CAD build for the part. Positions are in the model's coordinates, mm. Give positions to 0.01 mm unless a question says otherwise; leave off trailing zeros. Loops run counter-clockwise (first coordinate to the right, second up) from the corner with the lowest first, then second, coordinate; pieces in that order, holes last.
Autodesk Inventor part; units mm, degrees
ref_plane "YZ Plane" through (0, 0, 0) normal (1, 0, 0) x (0, 1, 0)
ref_plane "XZ Plane" through (0, 0, 0) normal (0, 1, 0) x (-1, 0, 0)
ref_plane "XY Plane" through (0, 0, 0) normal (0, 0, 1) x (1, 0, 0)
sketch "Sketch1" plane through (0, 0, 0) normal (0, 0, 1) x (1, 0, 0)
  line L0 (-76.2, 25.4) -> (76.2, 25.4) construction
  line L1 (76.2, 25.4) -> (76.2, -25.4) construction
  line L2 (76.2, -25.4) -> (-76.2, -25.4) construction
  line L3 (-76.2, -25.4) -> (-76.2, 25.4) construction
  line L4 (-76.2, 25.4) -> (76.2, -25.4) construction
  line L5 (76.2, 25.4) -> (-76.2, -25.4) construction
  line L6 (63.5, 17.4625) -> (63.5, -17.4625) construction
  line L7 (9.525, 15.875) -> (41.275, 15.875) construction
  line L8 (41.275, 15.875) -> (41.275, -15.875) construction
  line L9 (41.275, -15.875) -> (9.525, -15.875) construction
  line L10 (9.525, -15.875) -> (9.525, 15.875) construction
  line L11 (9.525, 15.875) -> (41.275, -15.875) construction
  line L12 (41.275, 15.875) -> (9.525, -15.875) construction
  line L13 (76.2, 101.6) -> (187.452, 101.6) construction
  line L14 (187.452, 101.6) -> (187.452, -25.4) construction
  line L15 (187.452, -25.4) -> (76.2, -25.4) construction
  line L16 (76.2, -25.4) -> (76.2, 101.6) construction
  line L17 (76.2, 101.6) -> (187.452, -25.4) construction
  line L18 (187.452, 101.6) -> (76.2, -25.4) construction
  point P0 (0, 0)
  point P1 (63.5, 0)
  point P2 (25.4, 0)
  point P3 (50.8, 0)
  point P4 (0, 0)
  point P5 (9.525, 0)
  point P6 (-12.7, 17.4625)
  point P7 (-12.7, -17.4625)
  point P8 (-25.4, 0)
  point P9 (-38.1, 17.4625)
  point P10 (-38.1, -17.4625)
  point P11 (-50.8, 0)
  point P12 (-63.5, 17.4625)
  point P13 (-63.5, -17.4625)
  point P14 (131.826, 38.1)
  dimension "d0" = 152.4
  dimension "d1" = 50.8
  dimension "d2" = 34.925
  dimension "d3" = 12.7
  dimension "d4" = 31.75
  dimension "d5" = 31.75
  dimension "d6" = 34.925
  dimension "d7" = 25.4
  dimension "d8" = 9.525
  dimension "d9" = 12.7
  dimension "d10" = 12.7
  dimension "d11" = 12.7
  dimension "d12" = 12.7
  dimension "d13" = 12.7
  dimension "d14" = 111.252
  dimension "d15" = 127
  dimension "d16" = 76.2
sketch "Sketch2" plane through (0, 0, 0) normal (0, 0, 1) x (1, 0, 0)
  line L0 (63.5, 17.4625) -> (63.5, -17.4625) construction
  line L1 (76.2, 25.4) -> (76.2, -25.4) construction
  line L2 (76.2, -25.4) -> (76.2, 101.6) construction
  line L3 (187.452, -25.4) -> (76.2, -25.4) construction
  line L4 (187.452, 101.6) -> (187.452, -25.4) construction
  line L5 (76.2, 101.6) -> (187.452, -25.4) construction
  line L6 (187.452, 101.6) -> (76.2, -25.4) construction
  line L7 (76.2, 101.6) -> (187.452, 101.6) construction
  line L8 (9.525, 15.875) -> (41.275, 15.875) construction
  line L9 (41.275, 15.875) -> (41.275, -15.875) construction
  line L10 (41.275, -15.875) -> (9.525, -15.875) construction
  line L11 (9.525, -15.875) -> (9.525, 15.875) construction
  line L12 (9.525, 15.875) -> (41.275, -15.875) construction
  line L13 (41.275, 15.875) -> (9.525, -15.875) construction
  line L14 (-76.2, 25.4) -> (76.2, 25.4) construction
  line L15 (76.2, -25.4) -> (-76.2, -25.4) construction
  line L16 (-76.2, 25.4) -> (76.2, -25.4) construction
  line L17 (76.2, 25.4) -> (-76.2, -25.4) construction
  line L18 (-76.2, -25.4) -> (-76.2, 25.4) construction
  line L19 (0, 25.4) -> (0, -25.4)
  line L20 (0, -25.4) -> (-76.2, -25.4)
  line L21 (-76.2, -25.4) -> (-76.2, 25.4)
  line L22 (-76.2, 25.4) -> (25.7652, 154.4619)
  circle A0 centre (44.45, 139.7) radius 14.2875
  circle A1 centre (44.45, 139.7) radius 23.8125 construction
  line L23 (68.2061, 141.338) -> (76.2, 25.4)
  line L24 (76.2, 25.4) -> (76.2, -25.4)
  line L25 (76.2, -25.4) -> (50.8, -25.4)
  line L26 (50.8, -25.4) -> (50.8, 25.4)
  line L27 (50.8, 25.4) -> (0, 25.4)
  arc A2 (68.2061, 141.338) -> (25.7652, 154.4619) centre (44.45, 139.7) ccw
  point P0 (0, 0)
  point P1 (63.5, 0)
  point P2 (131.826, 38.1)
  point P3 (9.525, 0)
  point P4 (0, 0)
  point P5 (25.4, 0)
  point P6 (-63.5, -17.4625)
  point P7 (-63.5, 17.4625)
  point P8 (-50.8, 0)
  point P9 (-38.1, -17.4625)
  point P10 (-38.1, 17.4625)
  point P11 (-25.4, 0)
  point P12 (-12.7, -17.4625)
  point P13 (-12.7, 17.4625)
  point P14 (0, 0)
  point P15 (50.8, 0)
  point P16 (0, 0)
  dimension "d17" = 28.575
  dimension "d18" = 9.525
  dimension "d20" = 9.525
  dimension "d21" = 9.525
  dimension "d31" = 165.1
  dimension "d32" = 19.05
extrude "Extrusion1" add sketch "Sketch2" along normal blind 6.35
hole "Hole1" at (76.2, 101.6, 0) at (131.826, 38.1, 0) at (187.452, -25.4, 0) at (9.525, 0, 0) at (9.525, 15.875, 0) at (41.275, -15.875, 0) at (41.275, 15.875, 0) at (9.525, -15.875, 0) at (25.4, 0, 0) at (-63.5, -17.4625, 0) at (-63.5, 17.4625, 0) at (-50.8, 0, 0) at (-38.1, -17.4625, 0) at (-38.1, 17.4625, 0) at (-25.4, 0, 0) at (-12.7, -17.4625, 0) at (-12.7, 17.4625, 0) at (63.5, 17.4625, 0) at (63.5, -17.4625, 0) direction (0, 0, 1) diameter 5.1054 end through all
fillet "Fillet1" radius 3.175 7 edges at (50.8, 25.4, 3.175) (0, 25.4, 3.175) (0, -25.4, 3.175) (50.8, -25.4, 3.175) (76.2, -25.4, 3.175) (-76.2, -25.4, 3.175) (-76.2, 25.4, 3.175)
sketch "Sketch3" plane through (0, 0, 6.35) normal (0, 0, 1) x (1, 0, 0)
  circle A0 centre (63.5, 17.4625) radius 2.5527 construction
  circle A1 centre (-12.7, -17.4625) radius 2.5527 construction
  circle A2 centre (-38.1, 17.4625) radius 2.5527 construction
  circle A3 centre (-50.8, 0) radius 2.5527 construction
  circle A4 centre (-63.5, -17.4625) radius 2.5527 construction
  circle A5 centre (-63.5, 17.4625) radius 2.5527 construction
  circle A6 centre (-38.1, -17.4625) radius 2.5527 construction
  circle A7 centre (-25.4, 0) radius 2.5527 construction
  circle A8 centre (-12.7, 17.4625) radius 2.5527 construction
  circle A9 centre (63.5, -17.4625) radius 2.5527 construction
  circle A10 centre (44.45, 139.7) radius 14.2875 construction
  arc A11 (68.2061, 141.338) -> (25.7652, 154.4619) centre (44.45, 139.7) ccw construction
  line L0 (68.2061, 141.338) -> (76.2, 25.4) construction
  line L1 (76.2, 25.4) -> (76.2, -22.225) construction
  arc A12 (73.025, -25.4) -> (76.2, -22.225) centre (73.025, -22.225) ccw construction
  line L2 (73.025, -25.4) -> (53.975, -25.4) construction
  arc A13 (50.8, -22.225) -> (53.975, -25.4) centre (53.975, -22.225) ccw construction
  line L3 (50.8, -22.225) -> (50.8, 22.225) construction
  arc A14 (50.8, 22.225) -> (47.625, 25.4) centre (47.625, 22.225) ccw construction
  line L4 (47.625, 25.4) -> (3.175, 25.4) construction
  arc A15 (3.175, 25.4) -> (0, 22.225) centre (3.175, 22.225) ccw construction
  line L5 (0, 22.225) -> (0, -22.225) construction
  arc A16 (-3.175, -25.4) -> (0, -22.225) centre (-3.175, -22.225) ccw construction
  line L6 (-3.175, -25.4) -> (-73.025, -25.4) construction
  arc A17 (-76.2, -22.225) -> (-73.025, -25.4) centre (-73.025, -22.225) ccw construction
  line L7 (-76.2, -22.225) -> (-76.2, 24.2971) construction
  arc A18 (-75.5163, 26.2654) -> (-76.2, 24.2971) centre (-73.025, 24.2971) ccw construction
  line L8 (-75.5163, 26.2654) -> (25.7652, 154.4619) construction
  circle A19 centre (44.45, 139.7) radius 20.6375 construction
  line L9 (69.85, 25.1813) -> (61.8711, 140.9012) construction
  arc A20 (61.8711, 140.9012) -> (30.7478, 150.5254) centre (44.45, 139.7) ccw construction
  line L10 (30.7478, 150.5254) -> (-69.85, 23.1943) construction
  line L11 (-69.85, 23.1943) -> (-69.85, -19.05) construction
  line L12 (-69.85, -19.05) -> (-6.35, -19.05) construction
  line L13 (-6.35, -19.05) -> (-6.35, 22.225) construction
  arc A21 (3.175, 31.75) -> (-6.35, 22.225) centre (3.175, 22.225) ccw construction
  line L14 (3.175, 31.75) -> (47.625, 31.75) construction
  arc A22 (57.15, 22.225) -> (47.625, 31.75) centre (47.625, 22.225) ccw construction
  line L15 (57.15, 22.225) -> (57.15, -19.05) construction
  line L16 (57.15, -19.05) -> (69.85, -19.05) construction
  line L17 (69.85, -19.05) -> (69.85, 25.1813) construction
  line L18 (3.175, 31.75) -> (-63.0905, 31.75) construction
  line L19 (47.625, 31.75) -> (69.3971, 31.75) construction
  circle A23 centre (-38.1, 17.4625) radius 2.5527 construction
  line L20 (-38.1, 17.4625) -> (44.45, 139.7) construction
  circle A24 centre (63.5, 17.4625) radius 2.5527 construction
  line L21 (63.5, 17.4625) -> (-19.5511, 86.8598) construction
  line L22 (65.8606, 83.0413) -> (-1.4492, 71.7339) construction
  line L23 (65.6411, 86.2239) -> (5.3247, 76.0913) construction
  line L24 (-24.6201, 31.75) -> (58.4936, 154.8223) construction
  line L25 (-32.2825, 31.75) -> (30.4064, 124.5777) construction
  line L26 (41.4499, 31.75) -> (-21.5201, 84.3676) construction
  line L27 (51.353, 31.75) -> (-17.5821, 89.3521) construction
  line L28 (66.08, 79.8586) -> (5.8815, 69.7459) construction
  line L29 (65.6411, 86.2239) -> (5.3247, 76.0913)
  line L30 (5.3247, 76.0913) -> (35.6688, 121.0239)
  line L31 (65.6411, 86.2239) -> (62.6277, 129.9287)
  arc A25 (35.6688, 121.0239) -> (62.6277, 129.9287) centre (44.45, 139.7) ccw
  line L32 (66.08, 79.8586) -> (5.8815, 69.7459)
  line L33 (5.8815, 69.7459) -> (51.353, 31.75)
  line L34 (51.353, 31.75) -> (69.3971, 31.75)
  line L35 (69.3971, 31.75) -> (66.08, 79.8586)
  line L36 (41.4499, 31.75) -> (-24.6201, 31.75)
  line L37 (-24.6201, 31.75) -> (-0.7863, 67.0424)
  line L38 (-0.7863, 67.0424) -> (41.4499, 31.75)
  line L39 (30.4064, 124.5777) -> (-2.1121, 76.4254)
  line L40 (-2.1121, 76.4254) -> (-17.5821, 89.3521)
  line L41 (-17.5821, 89.3521) -> (23.9296, 141.8953)
  arc A26 (23.9296, 141.8953) -> (30.4064, 124.5777) centre (44.45, 139.7) ccw
  line L42 (-21.5201, 84.3676) -> (-5.6845, 71.1354)
  line L43 (-5.6845, 71.1354) -> (-32.2825, 31.75)
  line L44 (-32.2825, 31.75) -> (-63.0905, 31.75)
  line L45 (-63.0905, 31.75) -> (-21.5201, 84.3676)
  point P0 (0, 0)
  dimension "d34" = 6.35
  dimension "d35" = 6.35
  dimension "d36" = 3.175
  dimension "d37" = 3.175
  dimension "d38" = 3.175
  dimension "d39" = 3.175
  dimension "d40" = 3.175
  dimension "d41" = 3.175
extrude "Extrusion2" cut sketch "Sketch3" against normal through all
fillet "Fillet2" radius 3.302 19 edges at (-21.5201, 84.3676, 3.175) (-63.0905, 31.75, 3.175) (-32.2825, 31.75, 3.175) (-5.6845, 71.1354, 3.175) (-0.7863, 67.0424, 3.175) (-24.6201, 31.75, 3.175) (41.4499, 31.75, 3.175) (30.4064, 124.5777, 3.175) (23.9296, 141.8953, 3.175) (-17.5821, 89.3521, 3.175) (-2.1121, 76.4254, 3.175) (66.08, 79.8586, 3.175) (5.8815, 69.7459, 3.175) (51.353, 31.75, 3.175) (69.3971, 31.75, 3.175) (65.6411, 86.2239, 3.175) (62.6277, 129.9287, 3.175) (35.6688, 121.0239, 3.175) (5.3247, 76.0913, 3.175)
equation "\"d34\" = off"
equation "\"d35\" = off"
equation "\"d36\" = 0.5 * off"
equation "\"d37\" = 0.5 * off"
equation "\"d38\" = 0.5 * off"
equation "\"d39\" = 0.5 * off"
equation "\"d40\" = 0.5 * off"
equation "\"d41\" = 0.5 * off"
equation "\"off\" = 6.35"
properties part number "CL3-004" material "Aluminum 6061"
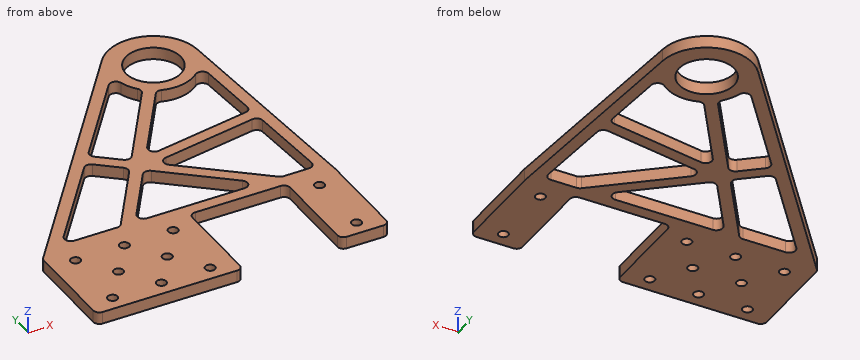
1. Saw through at A-A, the plane y = 5.5. List the corners of the cut face in (x, z).
Responses:
outline: (-76.2, 0) - (0, 0) - (0, 6.35) - (-76.2, 6.35) - close; (50.8, 0) - (76.2, 0) - (76.2, 6.35) - (50.8, 6.35) - close
2. Saw through at B-B, the plane x = -50.8. List the corners of the cut face in (y, z), and give its area (3 significant figures).
Responses:
outline: (-25.4, 0) - (-2.55, 0) - (-2.55, 6.35) - (-25.4, 6.35) - close; (2.55, 0) - (31.75, 0) - (31.75, 6.35) - (2.55, 6.35) - close; (47.31, 0) - (57.55, 0) - (57.55, 6.35) - (47.31, 6.35) - close
area: 396 mm2
3. Saw through at D-D, the plane x = 40. List the corners of the cut face in (y, z).
Responses:
outline: (25.4, 0) - (41.24, 0) - (41.24, 6.35) - (25.4, 6.35) - close; (75.48, 0) - (81.92, 0) - (81.92, 6.35) - (75.48, 6.35) - close; (119.55, 0) - (126.12, 0) - (126.12, 6.35) - (119.55, 6.35) - close; (153.28, 0) - (163.09, 0) - (163.09, 6.35) - (153.28, 6.35) - close
4. Probe line 1 along X through (y, z) = (36.5, 4); line 2 along Y through (x, z) = (-25.5, 5.5); line 3 along X through (y, z) = (102, 0.5). List the from-to ranges inside material, lowest first.
Responses:
line 1: x = -67.43 to -59.24, -29.07 to -21.37, 35.32 to 45.67, 69.07 to 75.43
line 2: y = -25.4 to -2.55, 2.55 to 41.79, 79.33 to 89.57
line 3: x = -15.68 to -7.59, 15.16 to 22.82, 64.55 to 70.92
5. Saw through at C-C, the plane y = 129. List the corners of the cut face in (x, z), and give its area (3 significant figures).
Responses:
outline: (5.65, 0) - (13.74, 0) - (13.74, 6.35) - (5.65, 6.35) - close; (26.8, 0) - (34.98, 0) - (34.98, 6.35) - (26.8, 6.35) - close; (53.92, 0) - (69.06, 0) - (69.06, 6.35) - (53.92, 6.35) - close
area: 199 mm2
6. Drop flat-ended pins along their axis: pin 1 (17 mm diameter, centred on x = 44.45, y = 139.7, fed in from -Z); pin 2 (3 mm diameter, centred on x = 59, z = 2.5, fed in from +Y); pin 3 (1 mm diameter, centred on x = -41, z = 5, fed in from +Y); pin 4 (1.9 mm diameter, centred on x = 6.5, z = 3, fed in from +Y). Give the stop position or say it passes through.
Responses:
pin 1: passes through
pin 2: stops at y = 159.62
pin 3: stops at y = 70.59
pin 4: stops at y = 131.28
